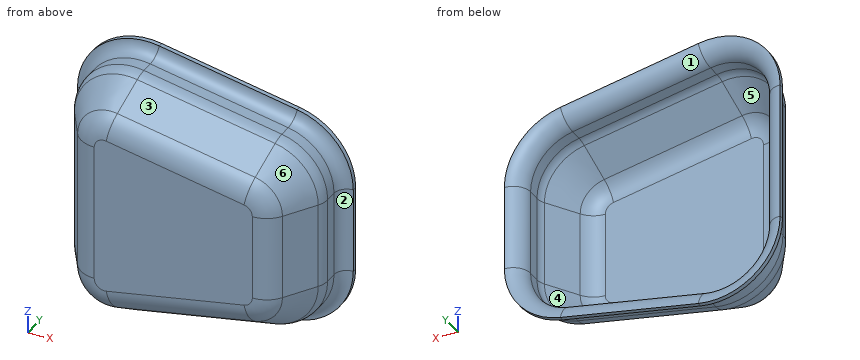
from build123d import *

# Parameters (mm, degrees)
BOSS_EXTRUDE2_START = 2.54
BOSS_EXTRUDE2_DEPTH = 2.54


with BuildPart() as part:
    # Sweep1: sweep along a path in Sketch3
    with BuildLine(Plane(origin=(0, 0, 0), x_dir=(1, 0, 0), z_dir=(0, 1, 0))) as sweep1_path:
        Line((-30.988229394, 75.53037161), (45.211770606, 61.05237161))
        ThreePointArc((45.211770606, 61.05237161), (67.44764437, 47.918620546), (76.2, 23.622))
        Line((76.2, 23.622), (76.2, -23.622))
        ThreePointArc((76.2, -23.622), (67.44764437, -47.918620546), (45.211770606, -61.05237161))
        Line((45.211770606, -61.05237161), (-30.988229394, -75.53037161))
        ThreePointArc((-30.988229394, -75.53037161), (-62.396620546, -67.44764437), (-76.2, -38.1))
        Line((-76.2, -38.1), (-76.2, 38.1))
        ThreePointArc((-76.2, 38.1), (-62.396620546, 67.44764437), (-30.988229394, 75.53037161))
    # Sketch2 → Sweep1 (sweep)
    with BuildSketch(Plane.XY):
        with BuildLine():
            Line((-66.675, 37.465), (-66.675, 30.734))
            ThreePointArc((-66.675, 30.734), (-66.304017394, 28.101588452), (-65.219967862, 25.674232841))
            Line((-65.219967862, 25.674232841), (-54.44795715, 8.493643788))
            ThreePointArc((-54.44795715, 8.493643788), (-49.836628957, 4.127648226), (-43.688, 2.54))
            Line((-43.688, 2.54), (-43.688, 0))
            ThreePointArc((-43.688, 0), (-51.066354749, 1.905177871), (-56.59994858, 7.144372546))
            Line((-56.59994858, 7.144372546), (-67.371959292, 24.324961599))
            ThreePointArc((-67.371959292, 24.324961599), (-68.745088699, 27.39961204), (-69.215, 30.734))
            Line((-69.215, 30.734), (-69.215, 37.465))
            ThreePointArc((-69.215, 37.465), (-71.260859133, 42.404140867), (-76.2, 44.45))
            Line((-76.2, 44.45), (-76.2, 46.99))
            ThreePointArc((-76.2, 46.99), (-69.464807909, 44.200192091), (-66.675, 37.465))
        make_face()
    sweep(path=sweep1_path.line)

    # Sketch5 → Boss-Extrude2 (add)
    with BuildSketch(Plane(origin=(0, 0, 0), x_dir=(1, 0, 0), z_dir=(0, 1, 0)).offset(BOSS_EXTRUDE2_START)):
        with BuildLine():
            Line((43.688, 23.622), (43.688, -23.622))
            ThreePointArc((43.688, -23.622), (42.404321174, -27.185504347), (39.143059689, -29.111787836))
            Line((39.143059689, -29.111787836), (-37.056940311, -43.589787836))
            ThreePointArc((-37.056940311, -43.589787836), (-41.663504347, -42.404321174), (-43.688, -38.1))
            Line((-43.688, -38.1), (-43.688, 0))
            Line((-43.688, 0), (-43.688, 38.1))
            ThreePointArc((-43.688, 38.1), (-41.663504347, 42.404321174), (-37.056940311, 43.589787836))
            Line((-37.056940311, 43.589787836), (39.143059689, 29.111787836))
            ThreePointArc((39.143059689, 29.111787836), (42.404321174, 27.185504347), (43.688, 23.622))
        make_face()
    extrude(amount=-BOSS_EXTRUDE2_DEPTH)


solid = part.part
Source: CAD feature listing. Evaluate the final solid. Frame: model axes, mm. Face numbers are marked on the shaded views. A direction names the side the tool comes from. Coordinates: 2 decimals unless noted, no trailing zeros. Order: outer loops, then holes, each group sorted by start corner. A loop starts at its lowest first (then second) coordinate and runs counter-clockwise, first axis right, second up.
Item 1: Cut plane A-A (y = 34). Return loops of the section in (x, z) (3 decimals).
Output values:
outline: (-69.215, -38.1) arc R31.115 ccw to (-32.292, -68.668) - (43.908, -54.19) arc R31.115 ccw to (69.215, -23.622) - (69.215, 23.622) arc R31.115 ccw to (43.908, 54.19) - (-32.292, 68.668) arc R31.115 ccw to (-69.215, 38.1) - close; hole (-66.675, -38.1) arc R28.575 ccw to (-32.766, -66.173) - (43.434, -51.695) arc R28.575 ccw to (66.675, -23.622) - (66.675, 23.622) arc R28.575 ccw to (43.434, 51.695) - (-32.766, 66.173) arc R28.575 ccw to (-66.675, 38.1) - close
Item 2: Cut plane C-C (y = 13.5). Return loops of the section in (x, z).
Output values:
outline: (-60.58, -38.1) arc R22.48 ccw to (-33.9, -60.19) - (42.3, -45.71) arc R22.48 ccw to (60.58, -23.62) - (60.58, 23.62) arc R22.48 ccw to (42.3, 45.71) - (-33.9, 60.19) arc R22.48 ccw to (-60.58, 38.1) - close; hole (-57.59, -38.1) arc R19.49 ccw to (-34.46, -57.24) - (41.74, -42.77) arc R19.49 ccw to (57.59, -23.62) - (57.59, 23.62) arc R19.49 ccw to (41.74, 42.77) - (-34.46, 57.24) arc R19.49 ccw to (-57.59, 38.1) - close
Item 3: Pull-direction query (Z, two-part tool) for the marked faces 1, 2, 3 and 4; classes: pulls with the +Z half, pulls with the -Z half, needs draft (parallel to the pull), parting line crosses it, or undercut.
Output values:
face 1: undercut
face 2: needs draft
face 3: pulls with the +Z half
face 4: undercut
Item 4: First-contact query: P1, Ø10, axis at x = -44, z = 59.5, coming from the -Y side; P2, Ø12, axis at y = 41, z = -45, coming from the +X side; P3, Ø1, axis at x = 32.5, y = 40.5, coming from the +Z side. Flat tips, straight axial feed; report the tip coordinate or a pass-through.
Output values:
P1: stops at y = 5.37
P2: stops at x = 72.46
P3: stops at z = 57.35
Item 5: Set-up query: the marked faces 5 and 6. Return all of +Z, -Z, +X, -X, +Y, -Y with unobstructed straight access to the full face (end or side cutting, diameter ignored); none if empty.
Output values:
face 5: +Y
face 6: +Z, +X, -Y
Item 6: Cut plane B-B (z = 0). Return loops of the section in (x, y) (3 decimals).
Output values:
outline: (-76.2, 44.45) arc R6.985 cw to (-69.215, 37.465) - (-69.215, 30.734) arc R12.065 ccw to (-67.372, 24.325) - (-56.6, 7.144) arc R15.24 ccw to (-43.688, 0) - (43.688, 0) arc R15.24 ccw to (56.6, 7.144) - (67.372, 24.325) arc R12.065 ccw to (69.215, 30.734) - (69.215, 37.465) arc R6.985 cw to (76.2, 44.45) - (76.2, 46.99) arc R9.525 ccw to (66.675, 37.465) - (66.675, 30.734) arc R9.525 cw to (65.22, 25.674) - (54.448, 8.494) arc R12.7 cw to (43.688, 2.54) - (-43.688, 2.54) arc R12.7 cw to (-54.448, 8.494) - (-65.22, 25.674) arc R9.525 cw to (-66.675, 30.734) - (-66.675, 37.465) arc R9.525 ccw to (-76.2, 46.99) - close
Item 7: Material intervals for line 1 (Z direction, x = -39, y = 35.5); line 2 (X direction, y = 35, z = 15) (3 decimals); line 3 (Z direction, x = -17, y = 15), sorted ascending.
Output values:
line 1: z = -69.2 to -66.66, 66.66 to 69.2
line 2: x = -69.215 to -66.675, 66.675 to 69.215
line 3: z = -57.94 to -54.88, 54.88 to 57.94
